Part model, mm, in its own coordinate system. Face numbers are marked on the shaded views. Coordinates: 2 decimals unless noted, no trailing zeros. Order: outer loops, then holes, each group sorted by start corner. A loop starts at its lowest first (then second) coordinate and runs counter-clockwise, first axis right, second up.
from build123d import *

# Parameters (mm, degrees)
F0_W     = 50
F0_H     = 50
F1_DEPTH = 12
F2_R     = 3
F3_DEPTH = 15
F4_R     = 3
F5_DEPTH = 15
F6_R     = 14
F7_DEPTH = 12.001


with BuildPart() as f1:
    # F0 (on Top) → F1 (new body)
    with BuildSketch(Plane.XY):
        with Locations((-5.501713, -4.568746)):
            Rectangle(F0_W, F0_H)
    extrude(amount=F1_DEPTH)

    # F2 (on face) → F3 (cut)
    with BuildSketch(Plane(origin=(-30.501713, 0, 0), x_dir=(0, -1, 0), z_dir=(-1, 0, 0))):
        with Locations((-10.431254, 6)):
            Circle(F2_R)
        with Locations((19.568746, 6)):
            Circle(F2_R)
    extrude(amount=-F3_DEPTH, mode=Mode.SUBTRACT)

    # F4 (on face) → F5 (cut)
    with BuildSketch(Plane.YZ.offset(19.498287)):
        with Locations((10.431254, 6)):
            Circle(F4_R)
        with Locations((-19.568746, 6)):
            Circle(F4_R)
    extrude(amount=-F5_DEPTH, mode=Mode.SUBTRACT)

    # F6 (on face) → F7 (cut, through all)
    with BuildSketch(Plane(origin=(0, 0, 0), x_dir=(1, 0, 0), z_dir=(0, 0, -1))):
        with Locations((-5.501713, 4.568746)):
            Circle(F6_R)
    extrude(amount=-F7_DEPTH, mode=Mode.SUBTRACT)


solid = f1.part
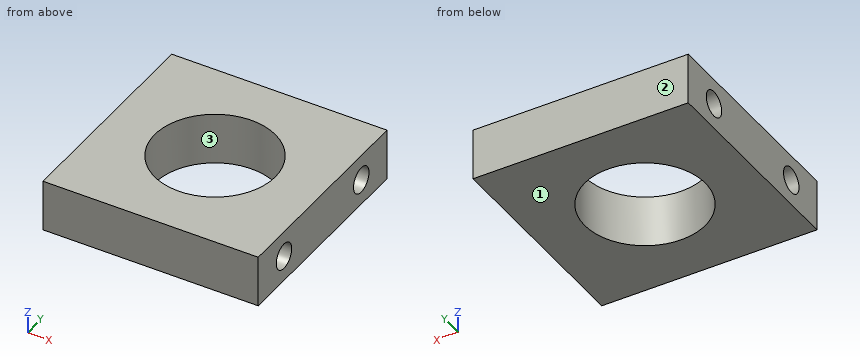
Q1. Cut at C-C on z = 6. Write the cut outline in (x, y), and give its area (3 significant figures).
Results list:
outline: (-30.5, -29.57) - (19.5, -29.57) - (19.5, -22.57) - (4.5, -22.57) - (4.5, -16.57) - (19.5, -16.57) - (19.5, 7.43) - (4.5, 7.43) - (4.5, 13.43) - (19.5, 13.43) - (19.5, 20.43) - (-30.5, 20.43) - (-30.5, 13.43) - (-15.5, 13.43) - (-15.5, 7.43) - (-30.5, 7.43) - (-30.5, -16.57) - (-15.5, -16.57) - (-15.5, -22.57) - (-30.5, -22.57) - close; hole circle Ø28 at (-5.5, -4.57)
area: 1,520 mm2
Q2. Wall check: line 1 along Y through (x, z) = (10, 7); line 2 along Y through (x, z) = (15.5, 6.75); line 3 along Z through (x, y) = (-18.5, 10.5). Give the ranges that are in metal, low to high.
Results list:
line 1: y = -29.57 to -22.4, -16.74 to 7.6, 13.26 to 20.43
line 2: y = -29.57 to -22.47, -16.66 to 7.53, 13.34 to 20.43
line 3: z = 0 to 3, 9 to 12
Q3. Pin check, flat tips, straight feed: pin 1 Ø1.8 at (y, z) = (-20, 6.5) entering from +X; pin 2 Ø1.8 at (y, z) = (10, 7) entering from -X. Stop position of each tip, or through.
Results list:
pin 1: stops at x = 4.5
pin 2: stops at x = -15.5
Q4. Mould opens along Y. For the marked faces 1, 2 and 3 say: pulls with the +Y half, pulls with the -Y half, needs draft (parallel to the pull), parting line crosses it, or undercut.
Results list:
face 1: needs draft
face 2: pulls with the +Y half
face 3: undercut
Q5. Cut at B-B on x = -5.5. Write the cut outline in (y, z), and give its area (3 significant figures).
Results list:
outline: (-29.57, 0) - (-18.57, 0) - (-18.57, 12) - (-29.57, 12) - close; (9.43, 0) - (20.43, 0) - (20.43, 12) - (9.43, 12) - close
area: 264 mm2
Q6. Cut at D-D on y = 6.5. Write the cut outline in (x, z), and give its area (3 significant figures).
Results list:
outline: (-30.5, 0) - (-14.07, 0) - (-14.07, 12) - (-30.5, 12) - close; (3.07, 0) - (19.5, 0) - (19.5, 12) - (3.07, 12) - close
area: 394 mm2
Q7. Cut at A-A on x = 14.5. Write the cut outline in (y, z), and give its area (3 significant figures).
Results list:
outline: (-29.57, 0) - (20.43, 0) - (20.43, 12) - (-29.57, 12) - close; hole circle Ø6 at (-19.57, 6); hole circle Ø6 at (10.43, 6)
area: 543 mm2
